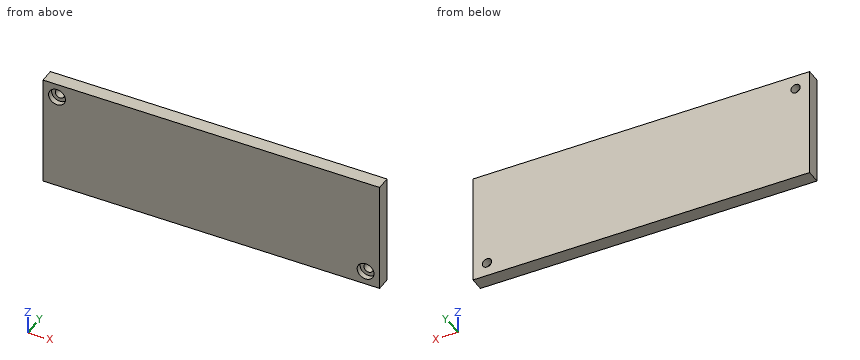
from build123d import *

# Parameters (mm, degrees)
F0_W           = 120
F0_H           = 40
F1_DEPTH       = 5
F3_D           = 3.3
F3_CBORE_D     = 6
F3_CBORE_DEPTH = 2


with BuildPart() as f1:
    # F0 (on Front) → F1 (new body)
    with BuildSketch(Plane.XZ):
        Rectangle(F0_W, F0_H)
    extrude(amount=F1_DEPTH)

    # F3 (through all)
    with Locations(Plane.XZ.offset(5)):
        with Locations((-55, 15), (55, -15)):
            CounterBoreHole(F3_D / 2, F3_CBORE_D / 2, F3_CBORE_DEPTH)


solid = f1.part
Build history of the part. All positions in model axes, mm. Round coordinates to 2 decimals unless told otherwise and drop trailing zeros. Loops run counter-clockwise (first coordinate to the right, second up) from the corner with the lowest first, then second, coordinate; pieces in that order, holes last. Notation, with made-up numbers: (75, 51.25) -> (85, 51.25) arc R21 cw to (85, 76.25) -> close; hole circle Ø4 at (33, 36.25). An arc over 180 degrees is marked (long way). Answer in a Markdown table with one row per item.
Item 1: Pin check, flat tips, straight feed: pin 1 (1.8 mm diameter, centred on x = 55.5, z = -15.5, fed in from -Y); pin 2 (5 mm diameter, centred on x = 55, z = -15, fed in from -Y). Stop position of each tip, or through.
Answers below:
| item | result |
|---|---|
| pin 1 | passes through |
| pin 2 | stops at y = -3 |
Item 2: Saw through at A-A (z = -15). Write the cut outline in (x, y), and give its area (3 significant figures).
Answers below:
| item | result |
|---|---|
| outline | (-60, -5) -> (52, -5) -> (52, -3) -> (53.35, -3) -> (53.35, 0) -> (-60, 0) -> close; (56.65, -3) -> (58, -3) -> (58, -5) -> (60, -5) -> (60, 0) -> (56.65, 0) -> close |
| area | 578 mm² |
Item 3: Drill centre lines: L1, parallel to Z at x = -55, y = -2.15; L2, parallel to Z at x = -55, y = -3.8; L3, parallel to X at y = -4.3, z = -13. Where is each one in solid material? Low to high. Write a range as [from, to].
Answers below:
| item | result |
|---|---|
| L1 | z = [-20, 13.35], [16.65, 20] |
| L2 | z = [-20, 12], [18, 20] |
| L3 | x = [-60, 52.76], [57.24, 60] |
Item 4: Saw through at B-B (x = 55). Write the cut outline in (y, z), and give its area (3 significant figures).
Answers below:
| item | result |
|---|---|
| outline | (-5, -20) -> (0, -20) -> (0, -16.65) -> (-3, -16.65) -> (-3, -18) -> (-5, -18) -> close; (-5, -12) -> (-3, -12) -> (-3, -13.35) -> (0, -13.35) -> (0, 20) -> (-5, 20) -> close |
| area | 178 mm² |
